Verification items for the finished model (mm, model axes). A direction names the side the tool comes from. Coordinates: 2 decimals unless noted, no trailing zeros. Write each loop counter-clockwise with the first axis right and the second up, starting at its lowest first coordinate (ties: lowest second). Pieces come first, ordered by that corner, then holes. Notation, with made-up numbers: M -9,-28.5 L 5,-28.5 A25 ccw 5,-3.5 Z; hole C 31,42.5 d8. An arc over 180 degrees is marked long. Answer in a Markdown table with one row per item.
from build123d import *

# Parameters (mm, degrees)
SKETCH1_W                      = 46
SKETCH1_H                      = 46
BOSS_EXTRUDE1_DEPTH            = 40
SKETCH2_W                      = 24
SKETCH2_H                      = 30
CUT_EXTRUDE1_DEPTH             = 56.181518645
SKETCH3_W                      = 15
SKETCH3_H                      = 10
SKETCH4_W                      = 15
SKETCH4_H                      = 10
SKETCH5_W                      = 22
SKETCH5_H                      = 15
SKETCH6_W                      = 22
SKETCH6_H                      = 15
F_15_0_15_DIAMETER_HOLE1_D     = 15
F_15_0_15_DIAMETER_HOLE1_DEPTH = 18
F_15_0_15_DIAMETER_HOLE2_D     = 15
F_15_0_15_DIAMETER_HOLE2_DEPTH = 66
F_15_0_15_DIAMETER_HOLE3_D     = 15
F_15_0_15_DIAMETER_HOLE3_DEPTH = 30
F_15_0_15_DIAMETER_HOLE4_D     = 15
F_15_0_15_DIAMETER_HOLE4_DEPTH = 84


with BuildPart() as part:
    # Sketch1 → Boss-Extrude1 (new body)
    with BuildSketch(Plane(origin=(-20, 0, 0), x_dir=(0, -1, 0), z_dir=(-1, 0, 0))):
        with Locations((0, -23)):
            Rectangle(SKETCH1_W, SKETCH1_H)
    extrude(amount=-BOSS_EXTRUDE1_DEPTH)

    # Sketch2 → Cut-Extrude1 (cut, through all)
    with BuildSketch(Plane(origin=(0, 0, -46), x_dir=(-1, 0, 0), z_dir=(0, 0, -1))):
        Rectangle(SKETCH2_W, SKETCH2_H)
    extrude(amount=-CUT_EXTRUDE1_DEPTH, mode=Mode.SUBTRACT)

    # Sketch3 → Revolve1 (revolve)
    with BuildSketch(Plane(origin=(0, 0, -23), x_dir=(-1, 0, 0), z_dir=(0, 0, -1)), mode=Mode.PRIVATE) as revolve1_sk:
        with Locations((-7.5, -28)):
            Rectangle(SKETCH3_W, SKETCH3_H)
    revolve(revolve1_sk.sketch.rotate(Axis((0, -33, -23), (0, 1, 0)), 270), axis=Axis((0, -33, -23), (0, 1, 0)))

    # Sketch4 → Revolve2 (revolve)
    with BuildSketch(Plane.XY.offset(-23), mode=Mode.PRIVATE) as revolve2_sk:
        with Locations((7.5, 28)):
            Rectangle(SKETCH4_W, SKETCH4_H)
    revolve(revolve2_sk.sketch.rotate(Axis((0, 33, -23), (0, -1, 0)), 270), axis=Axis((0, 33, -23), (0, -1, 0)))

    # Sketch5 → Revolve3 (revolve)
    with BuildSketch(Plane.XY.offset(-23)):
        with Locations((-31, 7.5)):
            Rectangle(SKETCH5_W, SKETCH5_H)
    revolve(axis=Axis((-42, 0, -23), (1, 0, 0)))

    # Sketch6 → Revolve4 (revolve)
    with BuildSketch(Plane(origin=(0, 0, -23), x_dir=(-1, 0, 0), z_dir=(0, 0, -1)), mode=Mode.PRIVATE) as revolve4_sk:
        with Locations((-31, 7.5)):
            Rectangle(SKETCH6_W, SKETCH6_H)
    revolve(revolve4_sk.sketch.rotate(Axis((42, 0, -23), (-1, 0, 0)), 180), axis=Axis((42, 0, -23), (-1, 0, 0)))

    # Ø15.0 (15) Diameter Hole1
    with Locations(Plane(origin=(0, -33, 0), x_dir=(-1, 0, 0), z_dir=(0, -1, 0))):
        with Locations((0, 23)):
            Hole(F_15_0_15_DIAMETER_HOLE1_D / 2, depth=F_15_0_15_DIAMETER_HOLE1_DEPTH)

    # Ø15.0 (15) Diameter Hole2
    with Locations(Plane(origin=(0, 33, 0), x_dir=(1, 0, 0), z_dir=(0, 1, 0))):
        with Locations((0, 23)):
            Hole(F_15_0_15_DIAMETER_HOLE2_D / 2, depth=F_15_0_15_DIAMETER_HOLE2_DEPTH)

    # Ø15.0 (15) Diameter Hole3
    with Locations(Plane.ZY.offset(42)):
        with Locations((-23, 0)):
            Hole(F_15_0_15_DIAMETER_HOLE3_D / 2, depth=F_15_0_15_DIAMETER_HOLE3_DEPTH)

    # Ø15.0 (15) Diameter Hole4
    with Locations(Plane(origin=(42, 0, 0), x_dir=(0, 0, -1), z_dir=(1, 0, 0))):
        with Locations((23, 0)):
            Hole(F_15_0_15_DIAMETER_HOLE4_D / 2, depth=F_15_0_15_DIAMETER_HOLE4_DEPTH)


solid = part.part
1) Depth check by flat-ended pin: pin 1 (2 mm diameter, centred on x = -33, y = 0.5, fed in from -Z); pin 2 (6 mm diameter, centred on y = -17, z = -20.5, fed in from -X); pin 3 (1.5 mm diameter, centred on x = -10.5, z = -40, fed in from -Y); pin 4 (13.5 mm diameter, centred on y = 0, z = -23, fed in from +X). Enter the tip coordinate at first touch or a pass-through.
Response values:
| item | result |
|---|---|
| pin 1 | stops at z = -38 |
| pin 2 | stops at x = -42 |
| pin 3 | stops at y = -23 |
| pin 4 | passes through |
2) Sectioned sample at D-D (z = -23). Give the number of separate pieces and of enclosed holes in the cut face, then the cut area to 3 significant figures.
Response values:
| item | result |
|---|---|
| separate pieces | 4 |
| enclosed holes | 0 |
| area | 1,600 mm² |
3) Sectioned sample at B-B (x = 0). Record the cut outline in (y, z).
Response values:
| item | result |
|---|---|
| outline | M -33,-38 L -23,-38 L -23,-46 L -15,-46 L -15,-30.5 L -33,-30.5 Z; M -33,-15.5 L -15,-15.5 L -15,0 L -23,0 L -23,-8 L -33,-8 Z; M 15,-46 L 23,-46 L 23,-38 L 33,-38 L 33,-30.5 L 15,-30.5 Z; M 15,-15.5 L 33,-15.5 L 33,-8 L 23,-8 L 23,0 L 15,0 Z |
4) Sectioned sample at C-C (y = -14). Record the cut outline in (x, z).
Response values:
| item | result |
|---|---|
| outline | M -42,-28.39 L -20,-28.39 L -20,-46 L -12,-46 L -12,0 L -20,0 L -20,-17.61 L -42,-17.61 Z; M 12,-46 L 20,-46 L 20,-28.39 L 42,-28.39 L 42,-17.61 L 20,-17.61 L 20,0 L 12,0 Z |
5) Tool access check on faces 1 (the face through (-30.846, -3.252, -37.643)), 2 (the face through (-12, -7, -18)), 3 (the face through (0.66, 28.07, -8.015)), 4 (the face through (30.846, 3.252, -37.643)). Record the directions out of +Z, -Z, +X, -X, +Y, -Y that give a thin tool (end or side, any length) a straight path to the whole face; none if there is none.
Response values:
| item | result |
|---|---|
| face 1 | -X |
| face 2 | +Z, -Z |
| face 3 | +Y |
| face 4 | +X |
6) Thickness scan on L1, parallel to X at y = -12.5, z = -32; L2, parallel to X at y = 4.5, z = -10.5; L3, parallel to Z at x = 0, y = -19.25. Record the ranges inside material, lowest first. Write a range as [from, to].
Response values:
| item | result |
|---|---|
| L1 | x = [-20, -12], [12, 20] |
| L2 | x = [-42, -12], [12, 42] |
| L3 | z = [-46, -30.5], [-15.5, 0] |
7) Sectioned sample at A-A (z = -5.5). Record the cut outline in (x, y), then the cut area to 3 significant figures.
Response values:
| item | result |
|---|---|
| outline | M -20,-23 L 20,-23 L 20,23 L -20,23 Z; hole M -12,-15 L 12,-15 L 12,15 L -12,15 Z |
| area | 1,120 mm² |
8) Release check for a two-part mould opening along Z. For faces 5 (the face through (26.79, 0.33, -30.493)), 6 (the face through (20, 0, -7)), 7 (the face through (-14, 0, -46)) record: +Z half, -Z half, draft (parallel to the pull), parting line (faces both ways), or undercut.
Response values:
| item | result |
|---|---|
| face 5 | undercut |
| face 6 | draft |
| face 7 | -Z half |
